Geometry: see drawing. Coordinates: mm, zero at the bounding-box minimum. Coordinates: 2 decimals unless noted, no trailing zeros. Order: outer loops, then holes, each group sorted by start corner. A loop starts at its lowest first (then second) coordinate and runs counter-clockwise, first axis right, second up. Notation, with made-up numbers: M 19.5,-13.75 L 68.5,-13.75 A26 ccw 68.5,12.25 Z; hole C -15,-39.75 d11. An arc over 180 degrees is marked long. One line per item, written item: value.
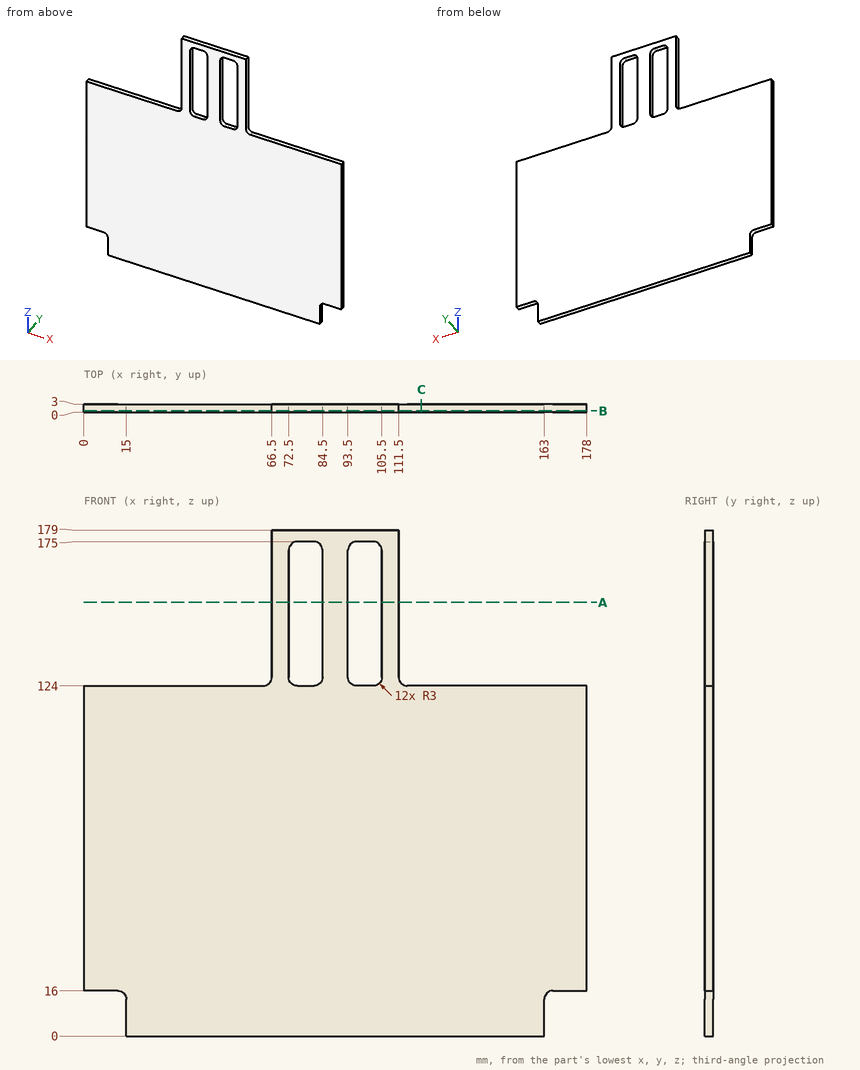
(1) Cut plane B-B on y = 0.6. Give the number of separate pieces and of enclosed holes in the cut face, plus the area to 3 significant figures.
Data:
separate pieces: 1
enclosed holes: 2
area: 22,900 mm2
(2) First-contact query: pin 1 (1.5 mm diameter, centred on y = 1.5, z = 159.5, fed in from -X); pin 2 (0.9 mm diameter, centred on x = 45.5, y = 1.5, fed in from +Z). Flat tips, straight axial feed; report the tip coordinate or a pass-through.
Data:
pin 1: stops at x = 66.5
pin 2: stops at z = 124
(3) Cut plane A-A on z = 153.5. Output: boundary loops of the cut face in (x, y).
Data:
outline: M 66.5,0 L 72.5,0 L 72.5,3 L 66.5,3 Z; M 84.5,0 L 93.5,0 L 93.5,3 L 84.5,3 Z; M 105.5,0 L 111.5,0 L 111.5,3 L 105.5,3 Z
(4) Ray query, line 1 (X direction, y = 1.3, z = 130.5); line 2 (Z direction, x = 102.5, y = 0.15); line 3 (Z direction, x = 40.5, y = 2.05). Return the intervals inside material, ascending. Write a range as from..to.
Data:
line 1: x = 66.5..72.5, 84.5..93.5, 105.5..111.5
line 2: z = 0..124, 175..179
line 3: z = 0..124
(5) Cut plane C-C on x = 119.5. Output: boundary loops of the cut face in (y, z), plus the area to 3 significant figures.
Data:
outline: M 0,0 L 3,0 L 3,124 L 0,124 Z
area: 372 mm2
